```python
from build123d import *

# Parameters (mm, degrees)
SKETCH_1_R             = 1.55
EXTRUDE_409_DEPTH      = 2.5
EXTRUDE_START          = 2.5
EXTRUDE_652_DEPTH      = 7.5
SKETCH_3_W             = 4.5
SKETCH_3_H             = 12.978713764
EXTRUDE_1_DEPTH        = 9.75
CHAMFER_1_SIZE         = 1
CUT_EXTRUDE_1251_DEPTH = 2
CUT_EXTRUDE_M3_REACH   = 27.038
SKETCH_6_R             = 1.55
EXTRUDE_1_2_DEPTH      = 7.25
CUT_EXTRUDE_1709_DEPTH = 26.037686694
EXTRUDE_START_2        = 1.5
SKETCH_8_R             = 1.55
EXTRUDE_2_DEPTH        = 1.5
FILLET_5_R             = 0.75
FILLET_6_R             = 0.25


with BuildPart() as part:
    # 草图1 → Extrude 409 (new body)
    with BuildSketch(Plane(origin=(0, 0, 0), x_dir=(1, 0, 0), z_dir=(0, 1, 0))):
        with BuildLine():
            Line((10.1243866, 13.845154317), (-6.15423406, 2.01804411))
            ThreePointArc((-6.15423406, 2.01804411), (-7.315700706, -5.315167685), (0.017511089, -6.476634331))
            Line((0.017511089, -6.476634331), (10.1243866, 0.866440553))
            Line((10.1243866, 0.866440553), (10.1243866, 13.845154317))
        make_face()
        with Locations(Location((0, 0, 0), (0, 0, 270))):
            Circle(SKETCH_1_R, mode=Mode.SUBTRACT)
    extrude(amount=EXTRUDE_409_DEPTH)

    # 草图2 → Extrude 652 (add)
    with BuildSketch(Plane(origin=(0, 0, 0), x_dir=(1, 0, 0), z_dir=(0, 1, 0)).offset(EXTRUDE_START)):
        Polygon((0.017511089, -6.476634331), (1.193081594, -8.09466832), (11.299957105, -0.751593436), (10.1243866, 0.866440553), align=None)
        Polygon((-7.329804565, 3.636078099), (0.809505765, 9.549633202), (1.98507627, 7.931599213), (-6.15423406, 2.01804411), align=None)
    extrude(amount=-EXTRUDE_652_DEPTH)

    # 草图3 → Extrude 1 (add)
    with BuildSketch(Plane(origin=(0, 0, 0), x_dir=(1, 0, 0), z_dir=(0, 1, 0))):
        with Locations((12.3743866, 7.355797435)):
            Rectangle(SKETCH_3_W, SKETCH_3_H)
    extrude(amount=EXTRUDE_1_DEPTH)

    # 倒角1
    chamfer_1_edges = [part.edges().sort_by_distance(p)[0] for p in [
        (0, 2.5, -1.55),
    ]]
    chamfer(chamfer_1_edges, length=CHAMFER_1_SIZE)

    # 草图5 → Cut-Extrude 1251 (cut)
    with BuildSketch(Plane.ZY.offset(-10.1243866)):
        Polygon((-4.151503441, 5.755), (-5.753650438, 8.53), (-8.957944432, 8.53), (-10.560091429, 5.755), (-8.957944432, 2.98), (-5.753650438, 2.98), align=None)
    extrude(amount=-CUT_EXTRUDE_1251_DEPTH, mode=Mode.SUBTRACT)

    # 草图6 → M3螺孔 (cut, up to next)
    with BuildSketch(Plane.ZY.offset(-10.1243866), mode=Mode.PRIVATE) as cut_extrude_m3_sk1:
        with Locations((-7.355797435, 5.755)):
            Circle(SKETCH_6_R)
    cut_extrude_m3_tool1 = extrude(cut_extrude_m3_sk1.sketch, amount=-CUT_EXTRUDE_M3_REACH, mode=Mode.PRIVATE) & part.part
    add(cut_extrude_m3_tool1.solids().sort_by_distance((10.124387, 5.755, -7.355797))[0], mode=Mode.SUBTRACT)

    # 草图7 → Extrude 1 2 (add)
    with BuildSketch(Plane(origin=(0, 0, 0), x_dir=(1, 0, 0), z_dir=(0, 1, 0)).offset(EXTRUDE_START)):
        Polygon((10.1243866, 13.845154317), (8.6243866, 12.755340525), (8.6243866, 0.866440553), (10.1243866, 0.866440553), align=None)
    extrude(amount=EXTRUDE_1_2_DEPTH)

    # 草图5<2> → Cut-Extrude 1709 (cut, through all)
    with BuildSketch(Plane.ZY.offset(-10.1243866)):
        Polygon((-4.151503441, 5.755), (-5.753650438, 8.53), (-8.957944432, 8.53), (-10.560091429, 5.755), (-8.957944432, 2.98), (-5.753650438, 2.98), align=None)
    extrude(amount=CUT_EXTRUDE_1709_DEPTH, mode=Mode.SUBTRACT)

    # 草图8 → 结构补强螺母位-2 (add)
    with BuildSketch(Plane.ZY.offset(-12.1243866).offset(EXTRUDE_START_2)):
        Polygon((-5.753650438, 2.98), (-4.151503441, 5.755), (-5.753650438, 8.53), (-8.957944432, 8.53), (-10.560091429, 5.755), (-8.957944432, 2.98), align=None)
        with Locations((-7.355797435, 5.755)):
            Circle(SKETCH_8_R, mode=Mode.SUBTRACT)
    extrude(amount=-EXTRUDE_2_DEPTH)

    # 圆角5
    fillet_5_edges = [part.edges().sort_by_distance(p)[0] for p in [
        (11.299957105, -1.25, 0.751593436),
        (1.193081594, -1.25, 8.09466832),
        (1.98507627, 1.25, -7.931599213),
        (-7.329804565, -1.25, -3.636078099),
        (0.809505765, -1.25, -9.549633202),
        (-6.15423406, 1.25, -2.01804411),
        (0.017511089, 1.25, 6.476634331),
    ]]
    fillet(fillet_5_edges, radius=FILLET_5_R)

    # 圆角6
    fillet_6_edges = [part.edges().sort_by_distance(p)[0] for p in [
        (10.1243866, 1.25, -0.866440553),
    ]]
    fillet(fillet_6_edges, radius=FILLET_6_R)


solid = part.part
```
Verification items for the finished model (mm, model axes). A direction names the side the tool comes from. Give positions to 0.01 mm unless a question says otherwise; leave off trailing zeros. Order: outer loops, then holes, each group sorted by start corner. A loop starts at its lowest first (then second) coordinate and runs counter-clockwise, first axis right, second up. Notation, with made-up numbers: (17.25, 74.25) -> (29.25, 74.25) arc R23 cw to (29.25, 85.25) -> close; hole circle Ø10 at (-18.75, 28.25). An arc over 180 degrees is marked (long way). One line per item, written item: value.
(1) Sectioned sample at D-D on x = 7.75. Record the cut outline in (y, z).
Final values:
outline: (-5, 0.86) -> (0, 0.86) -> (0, -12.12) -> (2.5, -12.12) -> (2.5, 3.33) -> (-5, 3.33) -> close
(2) Sectioned sample at C-C on z = 6. Record the cut outline in (x, y).
Final values:
outline: (-6.72, 0) -> (0.67, 0) -> (0.67, -5) -> (4.08, -5) -> (4.08, 2.5) -> (-6.72, 2.5) -> close
(3) Gauge pin test, flat ends, axial feed: pin 1 (4 mm diameter, centred on x = -5.5, z = -2.5, fed in from +Y); pin 2 (1.9 mm diameter, centred on y = 5.76, z = -7.36, fed in from +X); pin 3 (4 mm diameter, centred on x = 0, z = 0, fed in from +Y); pin 4 (3 mm diameter, centred on x = -5.5, z = -1.5, fed in from -Y). Record the tip position at first contact, or that the pin passes through.
Final values:
pin 1: y = 2.5
pin 2: through
pin 3: y = 1.95
pin 4: y = -5
(4) Scan lines: line 1 along Y through (x, z) = (2.75, -7.75); line 2 along X through (y, z) = (9.25, -12); line 3 along Y through (x, z) = (10, -1.5). Record each from-to range of solid material in increasing order. Write a range as [from, to].
Final values:
line 1: [0, 2.5]
line 2: [8.62, 14.62]
line 3: [0, 9.75]
(5) Sectioned sample at B-B on x = 12.25. Record the cut outline in (y, z) (3 decimals).
Final values:
outline: (0, -13.845) -> (9.75, -13.845) -> (9.75, -0.866) -> (0, -0.866) -> close; hole circle Ø3.1 at (5.755, -7.356)
(6) Draft check along Z on faces 1 (the face through (-0.005, 1.268, 6.756)), 2 (the face through (2.03, 1.23, -8.24)), 3 (the face through (-2.028, -2.465, -5.016)), 4 (the face through (8.624, 6, -4)). Enter one of: pulls with the +Z half, pulls with the -Z half, needs draft (parallel to the pull), parting line crosses it, or undercut.
Final values:
face 1: pulls with the +Z half
face 2: pulls with the -Z half
face 3: undercut
face 4: needs draft
(7) Tool access check on faces 5 (the face through (-7.377, 1.232, 5.229)), 6 (the face through (9.64, 7.16, -9.75)), 7 (the face through (-6.52, -2.03, -2.52)), 8 (the face through (1.613, -2.031, -8.444)). Record the directions out of +Z, -Z, +X, -X, +Y, -Y that give a thin tool (end or side, any length) a straight path to the whole face; none if there is none.
Final values:
face 5: +Y, -Y
face 6: -X
face 7: -X, -Y
face 8: -Z, -Y
(8) Sectioned sample at A-A on y = -1.25. Record the cut outline in (x, z).
Final values:
outline: (-6.89, -3.03) arc R0.75 ccw to (-6.72, -4.08) -> (0.2, -9.11) arc R0.75 ccw to (1.25, -8.94) -> (1.99, -7.93) -> (-6.15, -2.02) -> close; (0.02, 6.48) -> (10.12, -0.87) -> (10.86, 0.14) arc R0.75 ccw to (10.69, 1.19) -> (1.8, 7.65) arc R0.75 ccw to (0.75, 7.49) -> close
